Check sheet for the modelled part. Datum: model origin and axes. Units: mm. A direction names the side the tool comes from. Round coordinates to 2 decimals unless told otherwise and drop trailing zeros. Order: outer loops, then holes, each group sorted by start corner. A loop starts at its lowest first (then second) coordinate and runs counter-clockwise, first axis right, second up. Notation, with made-up numbers: (42, -3.5) -> (46, -3.5) arc R30 cw to (46, 32.5) -> close; hole circle Ø10 at (27, 73). An arc over 180 degrees is marked (long way). Answer in a Markdown table with one row per item. Add a question column.
1. Sectioned sample at A-A, the plane y = 2.5. Record the boundary of the cut face in (x, z), then the cut area to 3 significant figures.
2. Material ranges on L1, parallel to Z at x = -12, y = -1.75; L2, parallel to Z at x = 5, y = 8.5; L3, parallel to X at y = -6, z = 40.5, recorded low to high. Write a range as from..to.
3. Sectioned sample at C-C, the plane z = 6.5. Record the boundary of the cut face in (x, y).
4. Sectioned sample at D-D, the plane x = 10.5. Record the boundary of the cut face in (y, z).
5. Access from +Z, -Z, +X, -X, +Y, -Y to the whole of each face (thin tool, end or side, straight path). Record for faces 1 (the cylindrical face through (-0.291, 7.385, 38.535)), 2 (the flat face through (0, -6, -2)), 3 (the flat face through (0, 6, -2)).
6. Sectioned sample at B-B, the plane x = -2.5. Record the boundary of the cut face in (y, z), then the cut area to 3 significant figures.
7. Draft check along X on faces 4 (the cylindrical face through (-7.951, -4.305, 38.535)), 5 (the cylindrical face through (2.67, 4.19, 41.51)), 6 (the flat face through (0, -6, 41.07)). Enter one of: +X half, -X half, draft (parallel to the pull), parting line (faces both ways), or undercut.
8. Depth check by flat-ended pin: P1, Ø6, axis at x = -5, y = 2.5, coming from the +Z side; P2, Ø1.5, axis at x = 9, y = -0.5, coming from the +Z side; P3, Ø4, axis at x = -2.5, z = 3, coming from the +Y side. Enter the tip coordinate at first touch or a pass-through.
```python
from build123d import *
from build123d.topology import SkipClean

# Parameters (mm, degrees)
SKETCH1_R                    = 12.95
BOSS_EXTRUDE1_DEPTH          = 41.07
SKETCH2_R                    = 4.97
BOSS_EXTRUDE2_DEPTH          = 0.9
SKETCH3_R                    = 1.5
BOSS_EXTRUDE3_DEPTH          = 14.14
F_2_0_2_DIAMETER_HOLE1_D     = 2
F_2_0_2_DIAMETER_HOLE1_DEPTH = 5
F_2_0_2_DIAMETER_HOLE1_TIP   = 0.600860619
BOSS_EXTRUDE4_START          = 4
BOSS_EXTRUDE4_DEPTH          = 4


with BuildPart() as part:
    # Sketch1 → Boss-Extrude1 (new body)
    with BuildSketch(Plane.XY):
        Circle(SKETCH1_R)
    extrude(amount=BOSS_EXTRUDE1_DEPTH)

    # Sketch2 → Boss-Extrude2 (add)
    with BuildSketch(Plane.XY.offset(41.07)):
        Circle(SKETCH2_R)
    extrude(amount=BOSS_EXTRUDE2_DEPTH)

    # Sketch3 → Boss-Extrude3 (add)
    with BuildSketch(Plane.XY.offset(41.97)):
        with Locations(Location((0, 0, 0), (0, 0, 180))):
            Circle(SKETCH3_R)
    extrude(amount=BOSS_EXTRUDE3_DEPTH)

    # Ø2.0 (2) Diameter Hole1
    with Locations(Plane.XY.offset(41.07)):
        with Locations((-0.508072965, 8.361313231), (7.50309849, -3.724675843), (-6.99690151, -4.60576447)):
            Hole(F_2_0_2_DIAMETER_HOLE1_D / 2, depth=F_2_0_2_DIAMETER_HOLE1_DEPTH)
            with Locations((0, 0, -(F_2_0_2_DIAMETER_HOLE1_DEPTH + F_2_0_2_DIAMETER_HOLE1_TIP / 2))):  # 118° drill point
                Cone(0, F_2_0_2_DIAMETER_HOLE1_D / 2, F_2_0_2_DIAMETER_HOLE1_TIP, mode=Mode.SUBTRACT)

    # Sketch6 → Boss-Extrude4 (add)
    with SkipClean():  # the faces are left unmerged after this step: merging them gives an invalid solid
        with BuildSketch(Plane(origin=(0, 0, 0), x_dir=(-1, 0, 0), z_dir=(0, 0, -1)).offset(BOSS_EXTRUDE4_START)):
            with BuildLine():
                ThreePointArc((-11.476170964, 6), (-12.95, 0), (-11.476170964, -6))
                Line((-11.476170964, -6), (11.476170964, -6))
                ThreePointArc((11.476170964, -6), (12.576146349, -3.089181608), (12.95, 0))
                ThreePointArc((12.95, 0), (12.576146349, 3.089181608), (11.476170964, 6))
                Line((11.476170964, 6), (-11.476170964, 6))
            make_face()
        extrude(amount=-BOSS_EXTRUDE4_DEPTH)


solid = part.part
```
Answer key:
| question | item | result |
|---|---|---|
| 1 | outline | (-12.71, -4) -> (12.71, -4) -> (12.71, 41.07) -> (4.3, 41.07) -> (4.3, 41.97) -> (-4.3, 41.97) -> (-4.3, 41.07) -> (-12.71, 41.07) -> close |
| 1 | area | 1,150 mm² |
| 2 | L1 | z = -4..41.07 |
| 2 | L2 | z = 0..41.07 |
| 2 | L3 | x = -11.48..11.48 |
| 3 | outline | circle Ø25.9 at (0, 0) |
| 4 | outline | (-7.58, 0) -> (-6, 0) -> (-6, -4) -> (6, -4) -> (6, 0) -> (7.58, 0) -> (7.58, 41.07) -> (-7.58, 41.07) -> close |
| 5 | face 1 | +Z |
| 5 | face 2 | -Z, +X, -X, -Y |
| 5 | face 3 | -Z, +X, -X, +Y |
| 6 | outline | (-12.71, 0) -> (-6, 0) -> (-6, -4) -> (6, -4) -> (6, 0) -> (12.71, 0) -> (12.71, 41.07) -> (4.3, 41.07) -> (4.3, 41.97) -> (-4.3, 41.97) -> (-4.3, 41.07) -> (-12.71, 41.07) -> close |
| 6 | area | 1,100 mm² |
| 7 | face 4 | undercut |
| 7 | face 5 | parting line |
| 7 | face 6 | draft |
| 8 | P1 | stops at z = 41.97 |
| 8 | P2 | stops at z = 41.07 |
| 8 | P3 | stops at y = 12.94 |
